Autodesk Inventor part; units mm, degrees
ref_plane "Work Plane1" through (0, 0, 5.5563) normal (0, 0, 1) x (1, 0, 0)
ref_plane "YZ Plane" through (0, 0, 0) normal (1, 0, 0) x (0, 1, 0)
ref_plane "XZ Plane" through (0, 0, 0) normal (0, 1, 0) x (-1, 0, 0)
sketch "Sketch1" plane through (0, 0, 0) normal (0, 0, 1) x (1, 0, 0)
  line L0 (0, -10.9985) -> (-9.525, -5.4993)
  line L1 (-9.525, -5.4993) -> (-9.525, 5.4993)
  line L2 (-9.525, 5.4993) -> (0, 10.9985)
  line L3 (0, 10.9985) -> (9.525, 5.4993)
  line L4 (9.525, 5.4993) -> (9.525, -5.4993)
  line L5 (9.525, -5.4993) -> (0, -10.9985)
  point P0 (0, 0)
  point P1 (0, 0)
  dimension "d0" = 19.05
  dimension "d1" = 21.9971
sketch "Sketch2" plane through (0, 0, 0) normal (0, 0, 1) x (1, 0, 0)
  line L0 (-19.05, -19.05) -> (-19.05, 19.05)
  line L1 (-19.05, 19.05) -> (19.05, 19.05)
  line L2 (19.05, 19.05) -> (19.05, -19.05)
  line L3 (19.05, -19.05) -> (-19.05, -19.05)
  circle A0 centre (0, 0) radius 6.35 construction
  circle A1 centre (0, 0) radius 6.35 construction
  line L4 (0, -10.9985) -> (-9.525, -5.4993) construction
  line L5 (-9.525, -5.4993) -> (-9.525, 5.4993) construction
  line L6 (-9.525, 5.4993) -> (0, 10.9985) construction
  line L7 (0, 10.9985) -> (9.525, 5.4993) construction
  line L8 (9.525, 5.4993) -> (9.525, -5.4993) construction
  line L9 (9.525, -5.4993) -> (0, -10.9985) construction
  line L10 (0, 11.4027) -> (-9.875, 5.7013)
  line L11 (-9.875, 5.7013) -> (-9.875, -5.7013) construction
  line L12 (-9.875, -5.7013) -> (0, -11.4027) construction
  line L13 (0, -11.4027) -> (9.875, -5.7013) construction
  line L14 (9.875, -5.7013) -> (9.875, 5.7013) construction
  line L15 (9.875, 5.7013) -> (0, 11.4027)
  line L16 (-9.875, 5.7013) -> (-9.875, -19.05)
  line L17 (9.875, 5.7013) -> (9.875, -19.05)
  dimension "d11" = 38.1
  dimension "d12" = 0.35
extrude "Extrusion2" add sketch "Sketch2" along normal blind 11.1125 contours L0 L1 L2 L3 L17 L15 L10 L16
extrude "Extrusion4" add sketch "Sketch2" against normal blind 11.1125
ref_plane "Work Plane1" through (0, 0, 5.5563) normal (0, 0, 1) x (1, 0, 0)
mirror "Mirror1" about plane through (0, 0, 5.5563) normal (0, 0, 1) of "Extrusion4"
sketch "Sketch4" plane through (0, 0, -11.1125) normal (0, 0, -1) x (-1, 0, 0)
  point P0 (0, 0)
hole "Hole2" at (0, 0, -11.1125) direction (0, 0, 1) diameter 15.24 end through all
equation "\"d11\" = 2 * d0"
properties part number "halfinchNUT"
Design review of the part built by this model. Coordinates are the model's own, in mm. A direction names the side the tool comes from. Coordinates: 2 decimals unless noted, no trailing zeros. Order: outer loops, then holes, each group sorted by start corner. A loop starts at its lowest first (then second) coordinate and runs counter-clockwise, first axis right, second up. Notation, with made-up numbers: (-7.75, 51.5) -> (41.25, 51.5) arc R11 cw to (41.25, 55.5) -> close; hole circle Ø5 at (47, -20.75). An arc over 180 degrees is marked (long way). One line per item, written item: value. Start each with the question number.
Q1. Take a section at C-C, the plane x = -2. State the section outline as (y, z) points, then the cut area to 3 significant figures.
Q2. Mouldability with a two-part tool opening along Y and no side actions: class faces 3 (the flat face through (0, 19.05, 5)), 4 (the flat face through (19.05, 0, 5)), 5 (the cylindrical face through (7.44, -1.65, 16.75)) as pulls with the +Y half, pulls with the -Y half, needs draft (parallel to the pull), parting line crosses it, or undercut.
Q3. Tool access review of faces 1 (the flat face through (-4.87, 8.59, 5.48)), 2 (the cylindrical face through (7.44, -1.65, -5.48)): name each direction out of +Z, -Z, +X, -X, +Y, -Y from which nothing blocks a thin tool from reaching the whole face with its end or side.
Q4. Take a section at B-B, the plane z = 19. State the section outline as (x, y) points.
Q5. Insertion check: pin 1 Ø16 at (x, y) = (1.5, -6.5) entering from +Z. The pin has a flat end and moves straight along its axis. Give the tip position at first contact, or say it passes through.
Q6. For probe 1 along Y at (x, z) = (0, -5); probe 2 along Z at (x, y) = (6, -15.5), list the stretches that pass through material, from the lowest coordinate up.
Values follow:
1. outline: (-19.05, -11.11) -> (-7.35, -11.11) -> (-7.35, 0) -> (-19.05, 0) -> close; (-19.05, 11.11) -> (-7.35, 11.11) -> (-7.35, 22.23) -> (-19.05, 22.23) -> close; (7.35, -11.11) -> (19.05, -11.11) -> (19.05, 22.23) -> (7.35, 22.23) -> (7.35, 11.11) -> (10.25, 11.11) -> (10.25, 0) -> (7.35, 0) -> close
1. area: 618 mm2
2. face 3: pulls with the +Y half
2. face 4: needs draft
2. face 5: undercut
3. face 1: -Y
3. face 2: +Z, -Z
4. outline: (-19.05, -19.05) -> (19.05, -19.05) -> (19.05, 19.05) -> (-19.05, 19.05) -> close; hole circle Ø15.24 at (0, 0)
5. pin 1: stops at z = 22.23
6. probe 1: y = -19.05 to -7.62, 7.62 to 19.05
6. probe 2: z = -11.11 to 0, 11.11 to 22.23
